```python
from build123d import *

# Parameters (mm, degrees)
F1_DEPTH = 3.175
F3_DEPTH = 43.942
F5_DEPTH = 76.2
F6_DEPTH = 44.45


# Not quite as in the source:
# - a feature names something its author has since deleted; it is built from what else it names


with BuildPart() as f1:
    # F0 (on Front) → F1 (new body)
    with BuildSketch(Plane.XZ):
        Polygon((-34.925, -57.0107064), (9.4471751978, -57.0107064), (15.1238233026, -31.5280514049), (18.2228604819, -32.2184089652), (21.0519782071, -19.5184089652), (17.9529410277, -18.8280514049), (26.7166720978, 20.512617808), (29.8157092771, 19.8222602477), (32.5771395181, 32.2184089652), (29.4781023387, 32.9087665254), (34.8471751978, 57.0107064), (-34.925, 57.0107064), (-34.925, 31.6107064), (-38.1, 31.6107064), (-38.1, 18.9107064), (-34.925, 18.9107064), (-34.925, -18.9107064), (-38.1, -18.9107064), (-38.1, -31.6107064), (-34.925, -31.6107064), align=None)
    extrude(amount=F1_DEPTH)

    # F2 (on face) → F3 (join)
    with BuildSketch(Plane(origin=(-34.925, 0, 0), x_dir=(0, -1, 0), z_dir=(-1, 0, 0))):
        Polygon((0, -58.6279720227), (3.175, -57.0107064), (8.8332357394, -54.1285425744), (7.3921538265, -51.2994247047), (0, -55.0648030547), align=None)
    extrude(amount=-F3_DEPTH)

    # F4 (on face) → F5 (cut)
    with BuildSketch(Plane(origin=(-34.925, 0, 0), x_dir=(0, -1, 0), z_dir=(-1, 0, 0))):
        Polygon((0, 55.3934407773), (3.175, 57.0107064), (0, 57.0107064), align=None)
    extrude(amount=-F5_DEPTH, mode=Mode.SUBTRACT)

    # F2 (on face) → F6 (join)
    with BuildSketch(Plane(origin=(-34.925, 0, 0), x_dir=(0, -1, 0), z_dir=(-1, 0, 0))):
        Polygon((0, -58.6279720227), (3.175, -57.0107064), (8.8332357394, -54.1285425744), (7.3921538265, -51.2994247047), (0, -55.0648030547), align=None)
    extrude(amount=-F6_DEPTH)


solid = f1.part
```
Geometry check sheet. Reference: the model listing, model coordinates, mm. A direction names the side the tool comes from. Round coordinates to 2 decimals unless told otherwise and drop trailing zeros. Loops run counter-clockwise (first coordinate to the right, second up) from the corner with the lowest first, then second, coordinate; pieces in that order, holes last. Notation, with made-up numbers: (-3, 83.5) - (4, 83.5) arc R14 cw to (4, 90.5) - close; hole circle Ø2 at (34.5, 2.5). An arc over 180 degrees is marked (long way). Use a Markdown table: item, result.
Q1. Cross-section at B-B on y = -1.25. Record the cut outline in (x, z) (3 decimals).
Solutions:
| item | result |
|---|---|
| outline | (-38.1, -31.611) - (-34.925, -31.611) - (-34.925, -57.991) - (9.525, -57.991) - (9.525, -56.661) - (15.124, -31.528) - (18.223, -32.218) - (21.052, -19.518) - (17.953, -18.828) - (26.717, 20.513) - (29.816, 19.822) - (32.577, 32.218) - (29.478, 32.909) - (34.629, 56.03) - (-34.925, 56.03) - (-34.925, 31.611) - (-38.1, 31.611) - (-38.1, 18.911) - (-34.925, 18.911) - (-34.925, -18.911) - (-38.1, -18.911) - close |
Q2. Draft check along Z on faces 1 (the flat face through (-34.925, -2, -48)), 2 (the flat face through (22.273, -1.565, 0.567)), 3 (the flat face through (19.618, -1.565, -25.957)), 4 (the flat face through (-13.01, -8.12, -52.73)). Enter one of: released by +Z, released by -Z, zero draft, split by the parting line, or undercut.
Solutions:
| item | result |
|---|---|
| face 1 | zero draft |
| face 2 | undercut |
| face 3 | released by -Z |
| face 4 | released by +Z |
Q3. Access from +Z, -Z, +X, -X, +Y, -Y to the whole of each face (thin tool, end or side, straight path). Record for faces 5 (the flat face through (-13.01, -5.31, -52.36)), 6 (the flat face through (19.524, -1.565, -19.178)), 7 (the flat face through (-37, -2, -31.611)), 8 (the flat face through (9.525, -5, -55)), 9 (the flat face through (-34.925, -2, 44)).
Solutions:
| item | result |
|---|---|
| face 5 | +Z, +X, -X |
| face 6 | +X, +Y, -Y |
| face 7 | -Z, -X, +Y, -Y |
| face 8 | -Z, +X, -Y |
| face 9 | +Z, -X, +Y, -Y |
Q4. Cross-section at D-D on z = -21.5. Record the cut outline in (x, y) (3 decimals).
Solutions:
| item | result |
|---|---|
| outline | (-38.1, -3.175) - (20.611, -3.175) - (20.611, 0) - (-38.1, 0) - close |
Q5. Go/stop test with flat-tipped pins: P1, Ø1, axis at y = -2.5, z = -28.5, coming from the +X side; P2, Ø1.6, axis at x = -36, y = -1, coming from the -Z side; P3, Ø5, axis at x = 2.5, z = 44.5, coming from the -Y side (3 decimals). Record where each tip stops, or that it passes through.
Solutions:
| item | result |
|---|---|
| P1 | stops at x = 19.16 |
| P2 | stops at z = -31.61 |
| P3 | stops at y = -3.175 |
Q6. Material ranges on line 1 (Y direction, x = -5.5, z = -14) (3 decimals); line 2 (Z direction, x = 8.5, y = -2); line 3 (Z direction, x = 16, y = -0.5), recorded low to high.
Solutions:
| item | result |
|---|---|
| line 1 | y = -3.175 to 0 |
| line 2 | z = -57.61 to 56.41 |
| line 3 | z = -31.72 to 55.65 |
Q7. Cross-section at C-C on z = 44.5. Record the cut outline in (x, y) (3 decimals), plus the area to 3 significant figures.
Solutions:
| item | result |
|---|---|
| outline | (-34.925, -3.175) - (32.06, -3.175) - (32.06, 0) - (-34.925, 0) - close |
| area | 213 mm2 |
Q8. Cross-section at A-A on x = -9. Record the cut outline in (y, z) (3 decimals).
Solutions:
| item | result |
|---|---|
| outline | (-8.833, -54.129) - (0, -58.628) - (0, 55.393) - (-3.175, 57.011) - (-3.175, -53.448) - (-7.392, -51.299) - close |
